Geometry check sheet. Reference: the model listing, model coordinates, mm. A direction names the side the tool comes from. Give positions to 0.01 mm unless a question says otherwise; leave off trailing zeros. Loops run counter-clockwise (first coordinate to the right, second up) from the corner with the lowest first, then second, coordinate; pieces in that order, holes last. Notation, with made-up numbers: (-24, 76.5) -> (-18, 76.5) arc R25 cw to (-18, 90.5) -> close; hole circle Ø9 at (-17.75, 59.5). An arc over 180 degrees is marked (long way). Answer as a JSON object with one key per item and string values.
from build123d import *

# Parameters (mm, degrees)
BOSS_EXTRUDE1_DEPTH = 45.72
SKETCH2_W           = 0.35
SKETCH2_H           = 0.9


with BuildPart() as part:
    # Sketch1 → Boss-Extrude1 (new body, symmetric)
    with BuildSketch(Plane(origin=(0, 0, 0), x_dir=(1, 0, 0), z_dir=(0, 1, 0))):
        with BuildLine():
            Line((-2.236067977, 2), (2.236067977, 2))
            ThreePointArc((2.236067977, 2), (0, -3), (-2.236067977, 2))
        make_face()
    extrude(amount=BOSS_EXTRUDE1_DEPTH, both=True)

    # Sketch2 → Cut-Revolve1 (revolve, cut)
    with BuildSketch(Plane.XY):
        with Locations((2.825, 44.27)):
            Rectangle(SKETCH2_W, SKETCH2_H)
        with Locations((2.825, -44.27)):
            Rectangle(SKETCH2_W, SKETCH2_H)
    revolve(axis=Axis((0, 48.05613995, 0), (0, -1, 0)), mode=Mode.SUBTRACT)


solid = part.part
1) Depth check by flat-ended pin: P1, Ø1.5, axis at x = -2, y = 8, coming from the +Z side; P2, Ø1.5, axis at y = 17, z = 2, coming from the -X side. Enter the tip coordinate at first touch or a pass-through.
Geometry check:
{"P1": "stops at z = 2.73", "P2": "stops at x = -2.73"}
2) Material ranges on line 1 along Y through (x, z) = (1.9, 2.1); line 2 along X through (y, z) = (-40, 0.1); line 3 along Z through (x, y) = (0.1, -8), recorded low to high. Write a range as from..to.
Geometry check:
{"line 1": "y = -45.72..-44.72, -43.82..43.82, 44.72..45.72", "line 2": "x = -3..3", "line 3": "z = -2..3"}
3) Section check B-B on y = -16. Record the cut outline in (x, z).
Geometry check:
{"outline": "(-2.24, -2) -> (2.24, -2) arc R3 ccw (long way) to start"}
4) Tool access check on faces 4 (the face through (0, -45, 3)), 5 (the face through (0.09, -44.26, 2.65)). Record the directions out of +Z, -Z, +X, -X, +Y, -Y that give a thin tool (end or side, any length) a straight path to the whole face; none if there is none.
Geometry check:
{"face 4": "+Y, -Y", "face 5": "none"}
5) Section check A-A on z = 1.4. Record the cut outline in (x, y), plus the area to 3 significant figures.
Geometry check:
{"outline": "(-2.65, -45.72) -> (2.65, -45.72) -> (2.65, -44.72) -> (2.25, -44.72) -> (2.25, -43.82) -> (2.65, -43.82) -> (2.65, 43.82) -> (2.25, 43.82) -> (2.25, 44.72) -> (2.65, 44.72) -> (2.65, 45.72) -> (-2.65, 45.72) -> (-2.65, 44.72) -> (-2.25, 44.72) -> (-2.25, 43.82) -> (-2.65, 43.82) -> (-2.65, -43.82) -> (-2.25, -43.82) -> (-2.25, -44.72) -> (-2.65, -44.72) -> close", "area": "484 mm2"}
6) Draft check along Y on faces 1 (the face through (0.68, -43.82, 2.73)), 2 (the face through (0, 45.72, 0)), 3 (the face through (0, 1, -2)). Enter one of: pulls with the +Y half, pulls with the -Y half, needs draft (parallel to the pull), parting line crosses it, or undercut.
Geometry check:
{"face 1": "undercut", "face 2": "pulls with the +Y half", "face 3": "needs draft"}
